Input: part model. Units: mm. Frame: model coordinates. A direction names the side the tool comes from. Give positions to 0.01 mm unless a question says otherwise; leave off trailing zeros. Loops run counter-clockwise (first coordinate to the right, second up) from the corner with the lowest first, then second, coordinate; pieces in that order, holes last. Notation, with made-up numbers: (31.5, 46.5) -> (70.5, 46.5) arc R27 cw to (70.5, 84.5) -> close; hole circle Ø2 at (67.25, 65.25). An arc over 180 degrees is marked (long way). Use CSV: the item, a comma, the result in double quotes.
```python
from build123d import *

# Parameters (mm, degrees)
SKETCH1_W           = 114.3
SKETCH1_H           = 46.482
BOSS_EXTRUDE1_DEPTH = 3.175
SKETCH2_W           = 3.175
SKETCH2_H           = 38.1
CUT_EXTRUDE1_DEPTH  = 4.175


with BuildPart() as part:
    # Sketch1 → Boss-Extrude1 (new body)
    with BuildSketch(Plane.XY):
        with Locations((57.15, 23.241)):
            Rectangle(SKETCH1_W, SKETCH1_H)
    extrude(amount=BOSS_EXTRUDE1_DEPTH)

    # Sketch2 → Cut-Extrude1 (cut, through all)
    with BuildSketch(Plane.XY.offset(3.175)):
        with Locations((4.7625, 19.05)):
            Rectangle(SKETCH2_W, SKETCH2_H)
        with Locations((109.5375, 19.05)):
            Rectangle(SKETCH2_W, SKETCH2_H)
    extrude(amount=-CUT_EXTRUDE1_DEPTH, mode=Mode.SUBTRACT)


solid = part.part
```
1) Contact query for flat-ended pins moving along their axis: pin 1 (1 mm diameter, centred on x = 109, z = 2, fed in from -Y); pin 2 (1 mm diameter, centred on y = 23, z = 2.5, fed in from -X). Output: stop coordinate, or through.
From the geometry:
pin 1,"stops at y = 38.1"
pin 2,"stops at x = 0"
2) Mould query, pull axis X, two halves, no side actions, for faces 1 (the flat face through (56, 46.482, 2)), 2 (the flat face through (6.35, 19, 2)), 3 (the flat face through (110, 38.1, 2)), 4 (the flat face through (0, 23, 2)). Classes: pulls with the +X half, pulls with the -X half, needs draft (parallel to the pull), parting line crosses it, or undercut.
From the geometry:
face 1,"needs draft"
face 2,"undercut"
face 3,"undercut"
face 4,"pulls with the -X half"
3) Section query B-B (z = 0.95). Return loops of the section in (x, y) (3 decimals).
From the geometry:
outline,"(0, 0) -> (3.175, 0) -> (3.175, 38.1) -> (6.35, 38.1) -> (6.35, 0) -> (107.95, 0) -> (107.95, 38.1) -> (111.125, 38.1) -> (111.125, 0) -> (114.3, 0) -> (114.3, 46.482) -> (0, 46.482) -> close"
4) Reachability of faces 5 (the flat face through (5, 38.1, 2)), 6 (the flat face through (2, 0, 2)) from +Z, -Z, +X, -X, +Y, -Y: full face, straight path, thin tool, end or side. Return the list, or none.
From the geometry:
face 5,"+Z, -Z, -Y"
face 6,"+Z, -Z, +X, -X, -Y"
5) Ray query, line 1 (X direction, y = 13, z = 1.6) (3 decimals). Return the intervals inside material, ascending.
From the geometry:
line 1,"x = 0 to 3.175, 6.35 to 107.95, 111.125 to 114.3"
6) Section query A-A (y = 15). Return loops of the section in (x, z) (3 decimals).
From the geometry:
outline,"(0, 0) -> (3.175, 0) -> (3.175, 3.175) -> (0, 3.175) -> close; (6.35, 0) -> (107.95, 0) -> (107.95, 3.175) -> (6.35, 3.175) -> close; (111.125, 0) -> (114.3, 0) -> (114.3, 3.175) -> (111.125, 3.175) -> close"
